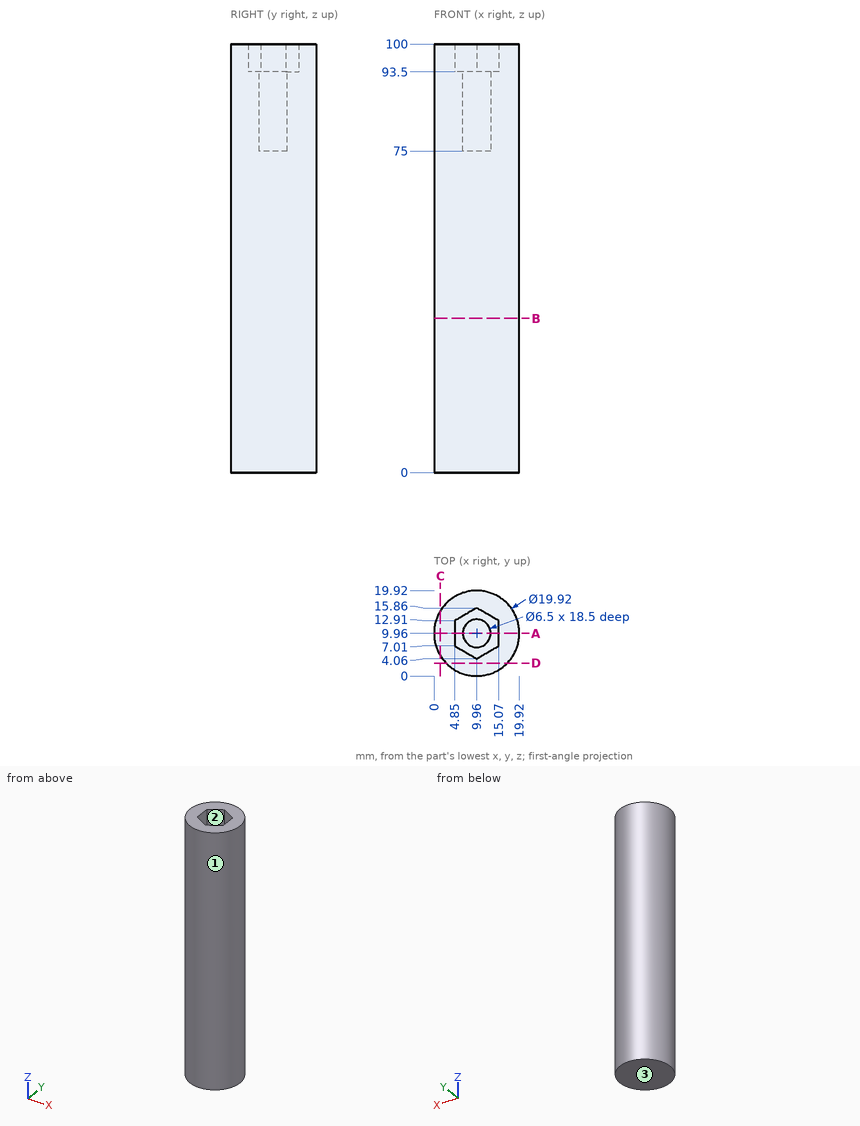
Can you work these out from the drawing? Everything is in mm from the part's minimum corner. Round coordinates to 2 decimals unless told otherwise and drop trailing zeros. Loops run counter-clockwise (first coordinate to the right, second up) from the corner with the lowest first, then second, coordinate; pieces in that order, holes last. Notation, with made-up numbers: (30.5, -21.5) -> (37.5, -21.5) arc R21 ccw to (37.5, 0.5) -> close; hole circle Ø4 at (52, 43). An arc over 180 degrees is marked (long way). One line per question, with ' | ' between items.
(1) If we section it at D-D on y = 3: List the corners of the cut face in (x, z) for me (1 decimal), and give its area (4 significant figures).
Model answer:
outline: (2.8, 0) -> (17.1, 0) -> (17.1, 100) -> (2.8, 100) -> close | area: 1,425 mm^2
(2) If I drill on probe 1 along Y at (x, z) = (9.96, 85.25); probe 2 along Z at (x, y) = (14.5, 12.25); probe 3 along X at (y, z) = (10.5, 35) (1 decimal), over which ranges is the centre line in solid material (lowest first)?
Model answer:
probe 1: y = 0 to 6.71, 13.21 to 19.92 | probe 2: z = 0 to 93.5 | probe 3: x = 0 to 19.9
(3) If we section it at C-C on x = 1.5: List the corners of the cut face in (y, z) for me, and give its area (3 significant figures).
Model answer:
outline: (4.7, 0) -> (15.22, 0) -> (15.22, 100) -> (4.7, 100) -> close | area: 1,050 mm^2
(4) For pin 1 Ø6 at (x, z) = (6.5, 14) entering from -Y; pin 2 Ø8.5 at (x, y) = (9.96, 9.96) entering from +Z; pin 3 Ø2 at (x, z) = (13, 45.5) entering from -Y, each with a flat end and sliding along its axis, tell me the tip position at first contact or that it passes through.
Model answer:
pin 1: stops at y = 0.01 | pin 2: stops at z = 93.5 | pin 3: stops at y = 0.21
(5) If we section it at A-A on y = 9.96: List the corners of the cut face in (x, z) for me.
Model answer:
outline: (0, 0) -> (19.92, 0) -> (19.92, 100) -> (15.07, 100) -> (15.07, 93.5) -> (13.21, 93.5) -> (13.21, 75) -> (6.71, 75) -> (6.71, 93.5) -> (4.85, 93.5) -> (4.85, 100) -> (0, 100) -> close
(6) If we section it at B-B on z = 36: List the corners of the cut face in (x, y) for me, and give its area (3 significant figures).
Model answer:
outline: circle Ø19.92 at (9.96, 9.96) | area: 312 mm^2
(7) Thinking about a two-plate mould opening in Y: for the marked faces 1, 2 and 3, which applies, released by +Y, released by -Y, zero draft, split by the parting line, or undercut?
Model answer:
face 1: split by the parting line | face 2: undercut | face 3: zero draft
